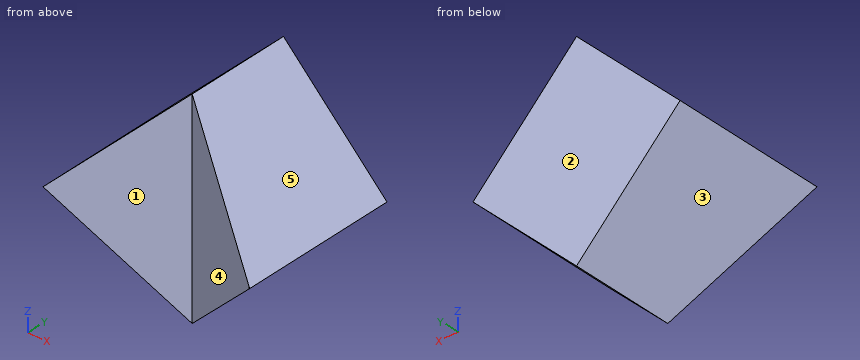
from build123d import *

# Parameters (mm, degrees)
F2_DEPTH = 30
F6_DEPTH = 61


with BuildPart() as f2:
    # F1 (on Front) → F2 (new body)
    with BuildSketch(Plane.XZ):
        Polygon((20, 0), (20, 40), (0, 20), align=None)
        Polygon((40, 20), (20, 40), (20, 0), align=None)
    extrude(amount=-F2_DEPTH)

    # F5 (on face) → F6 (cut)
    with BuildSketch(Plane.XY):
        Polygon((20, 10), (0, 0), (39.821261, 0), align=None)
    extrude(amount=F6_DEPTH, mode=Mode.SUBTRACT)


solid = f2.part
Here's how the part is built. I have some questions about the finished solid (model axes, mm). Face numbers are marked on the shaded views. A direction names the side the tool comes from. Coordinates: 2 decimals unless noted, no trailing zeros. Order: outer loops, then holes, each group sorted by start corner. A loop starts at its lowest first (then second) coordinate and runs counter-clockwise, first axis right, second up. Notation, with made-up numbers: M -25.75,77 L 23.25,77 A18 ccw 23.25,99 Z; hole C -29.75,-22 d1. An arc over 180 degrees is marked long. Answer as CSV lines item,"result". Start each with the question number.
1. I want a section at C-C, the plane z = 34. Write out the boundary of the cut face in (x, y), and give its area (3 significant figures).
2. On a 3-axis mill with a long thin cutter (end or side, diameter ignored), from which of +Z, -Z, +X, -X, +Y, -Y can I reach the whole of each face in a straight line? I mean the marked faces 4 and 5. Say none if no direction works.
3. I need wall thicknesses on line 1 (X direction, y = 6.75, z = 33); line 2 (X direction, y = 1.75, z = 19.5); line 3 (X direction, y = 21.5, z = 4). Which ranges of each line are inside material? Lowest first, please. Write a range as [from, to].
4. I want a section at A-A, the plane y = 4.25. Write out the boundary of the cut face in (x, z).
5. I want a section at D-D, the plane y = 19.5. Write out the boundary of the cut face in (x, z), and give its area (3 significant figures).
6. I want a section at B-B, the plane x = 16. Write out the boundary of the cut face in (y, z), and give its area (3 significant figures).
7. We'd pull the mould along X, two halves only. Please class the marked faces 1, 2 and 3: released by +X, released by -X, zero draft, split by the parting line, or undercut.
8. For pin 1 (1.5 mm diameter, centred on x = 31.5, z = 23.5, fed in from -Y); pin 2 (5 mm diameter, centred on y = 18, z = 32.5, fed in from -X); pin 3 (2 mm diameter, centred on x = 7, z = 10.5, fed in from -Y); pin 4 (6 mm diameter, centred on y = 15, z = 9, fed in from -X), each with a flat end and sliding along its axis, tell me the tip position at first contact or that it passes through.
Recorded:
1,outline,"M 14,7 L 20,10 L 26,6.97 L 26,30 L 14,30 Z"
1,area,"258 mm2"
2,face 4,"+Z, -Z, -Y"
2,face 5,"+Z, +X, +Y, -Y"
3,line 1,"x = [13, 13.5], [26.44, 27]"
3,line 2,"x = [0.5, 3.5], [36.35, 39.5]"
3,line 3,"x = [16, 24]"
4,outline,"M 0,20 L 8.5,11.5 L 8.5,28.5 Z; M 31.4,11.4 L 40,20 L 31.4,28.6 Z"
5,outline,"M 0,20 L 20,0 L 40,20 L 20,40 Z"
5,area,"800 mm2"
6,outline,"M 8,4 L 30,4 L 30,36 L 8,36 Z"
6,area,"704 mm2"
7,face 1,"undercut"
7,face 2,"zero draft"
7,face 3,"released by -X"
8,pin 1,"stops at y = 3.82"
8,pin 2,"stops at x = 10"
8,pin 3,"passes through"
8,pin 4,"stops at x = 8"
